Source: CAD feature listing. Evaluate the final solid. Frame: model axes, mm. A direction names the side the tool comes from. Round coordinates to 2 decimals unless told otherwise and drop trailing zeros. Write each loop counter-clockwise with the first axis right and the second up, starting at its lowest first coordinate (ties: lowest second). Pieces come first, ordered by that corner, then holes. Notation, with made-up numbers: (-2.5, -18.75) -> (53.5, -18.75) arc R28 ccw to (53.5, 17.25) -> close; hole circle Ø3 at (-1, 69.25). An arc over 180 degrees is marked (long way). Put each result on its own line as item: value.
```python
from build123d import *

# Parameters (mm, degrees)
BOSS_EXTRU_1_DEPTH      = 4
ESQUISSE2_R             = 3.5
ENL_V_MAT_EXTRU_1_DEPTH = 10
ENL_V_MAT_EXTRU_2_DEPTH = 2.5
ESQUISSE5_R             = 1.05
ENL_V_MAT_EXTRU_3_DEPTH = 59.124865591
ESQUISSE6_W             = 20
ESQUISSE6_H             = 10
BOSS_EXTRU_2_DEPTH      = 10
ESQUISSE7_W             = 15
ESQUISSE7_H             = 5
ENL_V_MAT_EXTRU_4_DEPTH = 10
CONG_2_R                = 1.5
CONG_3_R                = 15
ENL_V_START             = -20
ENL_V_MAT_EXTRU_5_DEPTH = 20


# Read off the part's stored shape, not the designer's step: Enlèv. mat.-Extru.5
with BuildPart() as part:
    # Esquisse1 → Boss.-Extru.1 (new body)
    with BuildSketch(Plane(origin=(0, 0, 0), x_dir=(0, 0, -1), z_dir=(1, 0, 0))):
        with BuildLine():
            Line((30, 5), (-30, 5))
            Line((-30, 5), (-30, -5))
            Line((-30, -5), (30, -5))
            Line((30, -5), (49.047311562, -7.439246248))
            ThreePointArc((49.047311562, -7.439246248), (57.484796152, -0.477311816), (50, 7.5))
            ThreePointArc((50, 7.5), (49.522688184, 7.484796152), (49.047311562, 7.439246248))
            Line((49.047311562, 7.439246248), (30, 5))
        make_face()
    extrude(amount=BOSS_EXTRU_1_DEPTH)

    # Esquisse2 → Enlèv. mat.-Extru.1 (cut)
    with BuildSketch(Plane(origin=(4, 0, 0), x_dir=(0, 0, -1), z_dir=(1, 0, 0))):
        with Locations((50, 0)):
            Circle(ESQUISSE2_R)
    extrude(amount=-ENL_V_MAT_EXTRU_1_DEPTH, mode=Mode.SUBTRACT)

    # Esquisse3 → Enlèv. mat.-Extru.2 (cut)
    with BuildSketch(Plane(origin=(4, 0, 0), x_dir=(0, 0, -1), z_dir=(1, 0, 0))):
        with BuildLine():
            Line((49.404376013, 3.448946515), (32.5, 2))
            ThreePointArc((32.5, 2), (30.5, 0), (32.5, -2))
            Line((32.5, -2), (49.404376013, -3.448946515))
            ThreePointArc((49.404376013, -3.448946515), (46.5, 0), (49.404376013, 3.448946515))
        make_face()
    extrude(amount=-ENL_V_MAT_EXTRU_2_DEPTH, mode=Mode.SUBTRACT)

    # Esquisse5 → Enlèv. mat.-Extru.3 (cut, through all)
    with BuildSketch(Plane(origin=(4, 0, 0), x_dir=(0, 0, -1), z_dir=(1, 0, 0))):
        with Locations((55.5, 0)):
            Circle(ESQUISSE5_R)
        with Locations((45.227029227, 4.772970773)):
            Circle(ESQUISSE5_R)
        with Locations(Location((45.227029227, -4.772970773, 0), (0, 0, 180))):
            Circle(ESQUISSE5_R)
    extrude(amount=-ENL_V_MAT_EXTRU_3_DEPTH, mode=Mode.SUBTRACT)

    # Esquisse6 → Boss.-Extru.2 (add)
    with BuildSketch(Plane.XY.offset(30)):
        with Locations((10, 0)):
            Rectangle(ESQUISSE6_W, ESQUISSE6_H)
    extrude(amount=BOSS_EXTRU_2_DEPTH)

    # Esquisse7 → Enlèv. mat.-Extru.4 (cut)
    with BuildSketch(Plane(origin=(0, 5, 0), x_dir=(1, 0, 0), z_dir=(0, 1, 0))):
        with Locations((10, -34.5)):
            Rectangle(ESQUISSE7_W, ESQUISSE7_H)
    extrude(amount=-ENL_V_MAT_EXTRU_4_DEPTH, mode=Mode.SUBTRACT)

    # Congé2
    cong_2_edges = [part.edges().sort_by_distance(p)[0] for p in [
        (2, -5, -30),
        (2, 5, -30),
        (20, 0, 40),
        (0, 0, 40),
        (20, 0, 30),
    ]]
    fillet(cong_2_edges, radius=CONG_2_R)

    # Congé3
    cong_3_edges = [part.edges().sort_by_distance(p)[0] for p in [
        (4, 0, 30),
    ]]
    fillet(cong_3_edges, radius=CONG_3_R)

    # Enlèv. mat.-Extru.5 outline → Enlèv. mat.-Extru.5 (cut)
    with BuildSketch(Plane(origin=(20, 0, 0), x_dir=(0, 0, -1), z_dir=(1, 0, 0)).offset(ENL_V_START)):
        Polygon((-40, 5), (-40, 4), (29.904343724, 5), align=None)
    extrude(amount=ENL_V_MAT_EXTRU_5_DEPTH, mode=Mode.SUBTRACT)


solid = part.part
```
Q1. Cut plane D-D on z = 3.5. Output: boundary loops of the cut face in (x, y).
Ans:
outline: (0, -5) -> (4, -5) -> (4, 4.52) -> (0, 4.52) -> close
Q2. Draft query along X for faces 1 (the flat face through (17.5, 0, 35)), 2 (the flat face through (4, 0, -21)), 3 (the flat face through (1.972, 6.243, -39.704)). Return one class per face: +X half, -X half, draft (parallel to the pull), parting line (faces both ways), or undercut.
Ans:
face 1: undercut
face 2: +X half
face 3: draft
Q3. Cut plane A-A on z = -55.5. Output: boundary loops of the cut face in (x, y).
Ans:
outline: (0, -5.1) -> (4, -5.1) -> (4, -1.05) -> (0, -1.05) -> close; (0, 1.05) -> (4, 1.05) -> (4, 5.1) -> (0, 5.1) -> close
Q4. Pin query (flat end, axial travel): pin 1 (2.5 mm diameter, centred on y = 4.77, z = -45.23, fed in from +X); pin 2 (2.5 mm diameter, centred on x = 6.5, y = 1.5, fed in from -Z); pin 3 (1 mm diameter, centred on x = 2.5, z = 21.5, fed in from -Y). Return the tip coordinate at first contact, or that it passes through.
Ans:
pin 1: stops at x = 4
pin 2: stops at z = 21
pin 3: stops at y = -5
Q5. Cut plane C-C on z = -22.5. Output: boundary loops of the cut face in (x, y).
Ans:
outline: (0, -5) -> (4, -5) -> (4, 4.89) -> (0, 4.89) -> close
Q6. Cut plane B-B on z = -35.5. Output: boundary loops of the cut face in (x, y), and give its area (3 significant figures).
Ans:
outline: (0, -5.7) -> (4, -5.7) -> (4, -2.26) -> (1.5, -2.26) -> (1.5, 2.26) -> (4, 2.26) -> (4, 5.7) -> (0, 5.7) -> close
area: 34.3 mm^2
Q7. Reachability of faces 4 (the flat face through (2.5, 0, 35)), 5 (the flat face through (3, -5, 13)), 6 (the flat face through (2.768, 2.735, -41.071)) from +Z, -Z, +X, -X, +Y, -Y: full face, straight path, thin tool, end or side. Return the list, or none.
Ans:
face 4: +Y, -Y
face 5: +Z, +X, -X, -Y
face 6: +X
Q8. Material intervals for line 1 (Y direction, x = 2.2, z = -50); line 2 (X direction, y = 3.25, z = 33); line 3 (X direction, y = -0.5, z = 6), sorted ascending. Write a range as [from, to].
Ans:
line 1: y = [-7.5, -3.5], [3.5, 7.5]
line 2: x = [0, 2.5], [17.5, 20]
line 3: x = [0, 4]
